Work out the finished part from the listing and answer in its coordinate system (mm). A direction names the side the tool comes from. Round coordinates to 2 decimals unless told otherwise and drop trailing zeros. Order: outer loops, then holes, each group sorted by start corner. A loop starts at its lowest first (then second) coordinate and runs counter-clockwise, first axis right, second up. Notation, with made-up numbers: (1, 41.5) - (18, 41.5) arc R8 cw to (18, 50.5) - close; hole circle Ø9 at (84.5, -23.75). An arc over 180 degrees is marked (long way). Use CSV: the item, a comma, the result in double quotes.
from build123d import *

# Parameters (mm, degrees)
F0_R     = 25
F1_DEPTH = 150.1
F2_R     = 30.985026
F2_R_2   = 25
F3_DEPTH = 25


with BuildPart() as f1:
    # F0 (on Front) → F1 (new body, symmetric)
    with BuildSketch(Plane.XZ):
        Circle(F0_R)
    extrude(amount=F1_DEPTH, both=True)

    # F2 (on Front) → F3 (join)
    with BuildSketch(Plane.XZ):
        Circle(F2_R)
        Circle(F2_R_2, mode=Mode.SUBTRACT)
    extrude(amount=F3_DEPTH)


solid = f1.part
(1) Each of these flat-tipped pins is pushed along its axis until it touches: pin 1 (1 mm diameter, centred on y = -8.5, z = 14, fed in from -X); pin 2 (6 mm diameter, centred on y = 105, z = -20, fed in from -X); pin 3 (1 mm diameter, centred on y = 109, z = 0, fed in from -X); pin 4 (5 mm diameter, centred on y = -13.5, z = 2, fed in from +X) (3 decimals). Where does it stop, or does it pass through?
Findings below:
pin 1,"stops at x = -27.89"
pin 2,"stops at x = -18.33"
pin 3,"stops at x = -25"
pin 4,"stops at x = 30.985"
(2) Find section B-B (x = 0). Determine the outline of the cut face in (y, z).
Findings below:
outline,"(-150.1, -25) - (-25, -25) - (-25, -30.99) - (0, -30.99) - (0, -25) - (150.1, -25) - (150.1, 25) - (0, 25) - (0, 30.99) - (-25, 30.99) - (-25, 25) - (-150.1, 25) - close"
(3) Find section A-A (z = 0). Determine the outline of the cut face in (x, y), and give its area (3 significant figures).
Findings below:
outline,"(-30.99, -25) - (-25, -25) - (-25, -150.1) - (25, -150.1) - (25, -25) - (30.99, -25) - (30.99, 0) - (25, 0) - (25, 150.1) - (-25, 150.1) - (-25, 0) - (-30.99, 0) - close"
area,"15,300 mm²"
(4) For faces 1 (the flat face through (-21, -25, 14)), 2 (the flat face through (0, -150.1, 0)), 3 (the flat face through (-21, 0, 14)), determine the directions among +Z, -Z, +X, -X, +Y, -Y from which every point of the face is accessible in a straight line to the end or side of a thin tool.
Findings below:
face 1,"-Y"
face 2,"+Z, -Z, +X, -X, -Y"
face 3,"+Y"
(5) Find the intervals of material crossed by L1, parallel to Y at x = 3, z = 28; L2, parallel to Z at x = -1, y = 19; L3, parallel to Z at x = 6, y = -27.5, in increasing order. Write a range as from..to.
Findings below:
L1,"y = -25..0"
L2,"z = -24.98..24.98"
L3,"z = -24.27..24.27"
(6) Find section C-C (y = -105). Determine the outline of the cut face in (x, z), and give its area (3 significant figures).
Findings below:
outline,"circle Ø50 at (0, 0)"
area,"1,960 mm²"
